Answer from the drawing. Dimensions are ordinates in mm from the lowest x, y and z of the part. A direction names the side the tool comes from. Coordinates: 2 decimals unless noted, no trailing zeros. Loops run counter-clockwise (first coordinate to the right, second up) from the corner with the lowest first, then second, coordinate; pieces in that order, holes last. Notation, with made-up numbers: (-39, -28.75) - (-2, -28.75) arc R35 cw to (-2, 5.25) - close; hole circle Ø9 at (50, -11). An arc over 180 degrees is marked (long way). Use one line per item in the form item = value. Start each with the question number.
1) A cutting plane is placed at B-B (x = 275.5). Give the vertices of the cut face in (y, z).
2) Each of these flat-tipped pins is pushed along its axis until it touches: P1, Ø23, axis at x = 165.5, y = 302, coming from the +Z side; P2, Ø1, axis at x = 51, z = 270.5, coming from the -Y side; P3, Ø10, axis at x = 98, y = 135, coming from the +Z side. Where does it stop, or does it pass through?
3) Consider line 1 (Z direction, x = 152, y = 140); line 2 (Y direction, x = 48.5, z = 260); line 3 (Y direction, x = 266, z = 47). Determine where each line is inside the solid, lowest interval first.
4) A cutting plane is placed at A-A (z = 19). Give the vertices of the cut face in (x, y), and give its area (3 significant figures).
5) A cutting plane is placed at D-D (x = 352). Give the vertices of the cut face in (y, z).
6) A cutting plane is placed at C-C (y = 73). Give the vertices of the cut face in (x, z).
7) Which of the six approach directions +Z, -Z, +X, -X, +Y, -Y give full straight-line access (tool end or side, diameter ignored) to the marked faces 1, 2, 3, 4 and 5?
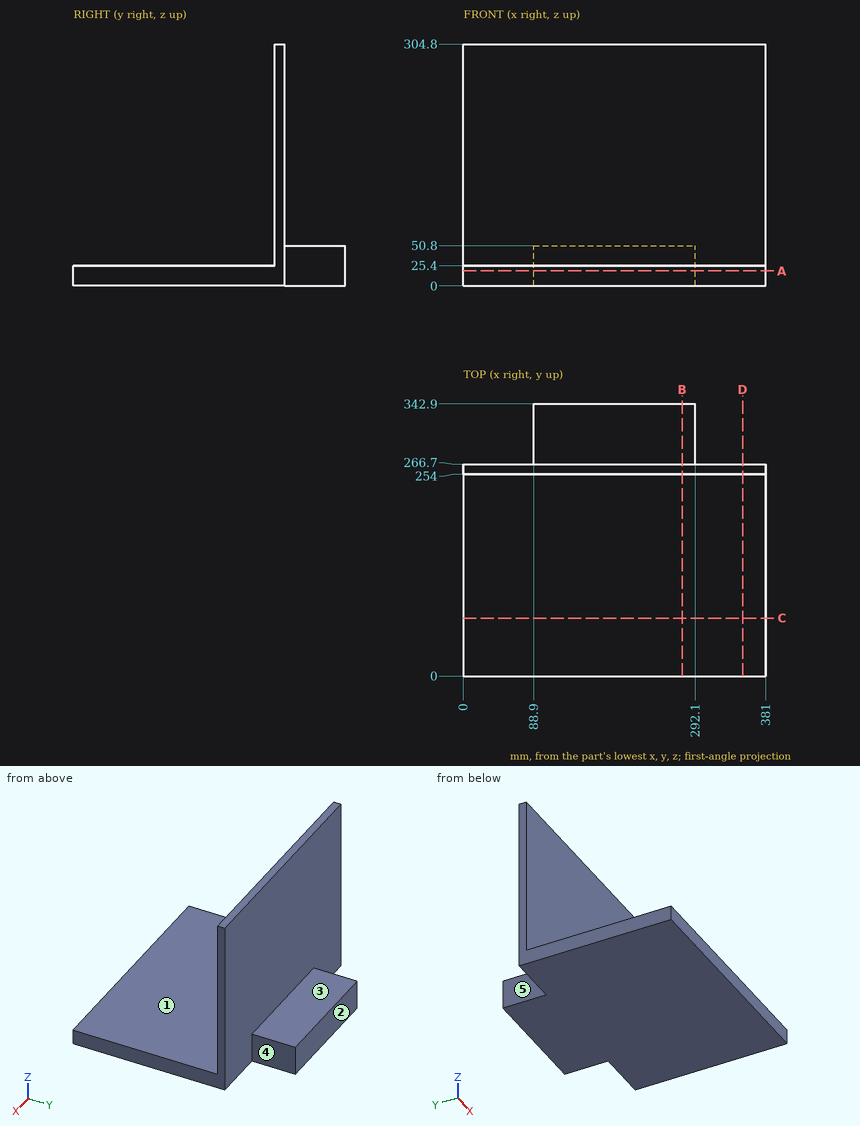
Found:
q1.outline = (0, 0) - (342.9, 0) - (342.9, 50.8) - (266.7, 50.8) - (266.7, 304.8) - (254, 304.8) - (254, 25.4) - (0, 25.4) - close
q2.P1 = 50.8
q2.P2 = 254
q2.P3 = 25.4
q3.line_1 = 0 to 25.4
q3.line_2 = 254 to 266.7
q3.line_3 = 254 to 342.9
q4.outline = (0, 0) - (381, 0) - (381, 266.7) - (292.1, 266.7) - (292.1, 342.9) - (88.9, 342.9) - (88.9, 266.7) - (0, 266.7) - close
q4.area = 117,000 mm^2
q5.outline = (0, 0) - (266.7, 0) - (266.7, 304.8) - (254, 304.8) - (254, 25.4) - (0, 25.4) - close
q6.outline = (0, 0) - (381, 0) - (381, 25.4) - (0, 25.4) - close
q7.face_1 = +Z, +X, -X, -Y
q7.face_2 = +Z, -Z, +X, -X, +Y
q7.face_3 = +Z, +X, -X, +Y
q7.face_4 = +Z, -Z, +X, +Y
q7.face_5 = +Z, -Z, -X, +Y
